```python
from build123d import *

# Parameters (mm, degrees)
F0_R     = 2.0955
F1_DEPTH = 6.35
F5_D     = 2.2606
F5_DEPTH = 5.08
F5_START = 0.1014065
F5_TIP   = 0.6791527577


with BuildPart() as f1:
    # F0 (on Top) → F1 (new body)
    with BuildSketch(Plane.XY):
        with BuildLine():
            ThreePointArc((-6.3375855209, 0.396875), (-0.1985345593, -6.3468956214), (6.35, 0))
            ThreePointArc((6.35, 0), (6.3468956214, 0.1985345593), (6.3375855209, 0.396875))
            ThreePointArc((6.3375855209, 0.396875), (0, 6.35), (-6.3375855209, 0.396875))
        make_face()
        Circle(F0_R, mode=Mode.SUBTRACT)
        with BuildLine():
            ThreePointArc((-6.3375855209, 0.396875), (0, 6.35), (6.3375855209, 0.396875))
            Line((6.3375855209, 0.396875), (0, 101.6))
            Line((0, 101.6), (-6.3375855209, 0.396875))
        make_face()
    extrude(amount=F1_DEPTH)

    # F5
    # its depths count from where the whole tool has entered the part; down to there all is cleared
    with Locations(Plane.XZ.offset(6.35).offset(-F5_START)):
        with Locations((0, 3.175)):
            Hole(F5_D / 2, depth=F5_DEPTH)
            with Locations((0, 0, -(F5_DEPTH + F5_TIP / 2))):  # 118° drill point
                Cone(0, F5_D / 2, F5_TIP, mode=Mode.SUBTRACT)


solid = f1.part
```
Geometry: final body of the model. Coordinates: model frame, mm. Coordinates: 2 decimals unless noted, no trailing zeros. Order: outer loops, then holes, each group sorted by start corner. A loop starts at its lowest first (then second) coordinate and runs counter-clockwise, first axis right, second up. Notation, with made-up numbers: (9, 89) -> (41, 89) arc R29 ccw to (41, 111) -> close; hole circle Ø5 at (12, -7). An arc over 180 degrees is marked (long way). Answer in a Markdown table with one row per item.
Item 1: Section B-B on x = 4.75. Output: boundary loops of the cut face in (y, z), plus the area to 3 significant figures.
Return value:
| item | result |
|---|---|
| outline | (-4.21, 0) -> (25.75, 0) -> (25.75, 6.35) -> (-4.21, 6.35) -> close |
| area | 190 mm² |
Item 2: Draft query along X for faces 1 (the flat face through (0, 36, 0)), 2 (the flat face through (3.213, 50.29, 3.131)), 3 (the flat face through (-3.124, 51.707, 3.131)), 4 (the cylindrical face through (1.13, -4.03, 3.22)). Return one class per face: released by +X, released by -X, zero draft, split by the parting line, or undercut.
Return value:
| item | result |
|---|---|
| face 1 | zero draft |
| face 2 | released by +X |
| face 3 | released by -X |
| face 4 | undercut |
Item 3: Contact query for flat-ended pins moving along their axis: P1, Ø5, axis at x = -3.5, y = 52.5, coming from the -Z side; P2, Ø1.4, axis at x = 0, z = 3.175, coming from the -Y side. Output: stop coordinate, or through.
Return value:
| item | result |
|---|---|
| P1 | stops at z = 0 |
| P2 | stops at y = 1.98 |
Item 4: Ray query, L1, parallel to X at y = 15.5, z = 0.5; L2, parallel to X at y = 18, z = 1.75. Return the intervals inside material, ascending.
Return value:
| item | result |
|---|---|
| L1 | x = -5.39 to 5.39 |
| L2 | x = -5.24 to 5.24 |
Item 5: Section A-A on y = 28.5. Output: boundary loops of the cut face in (x, z), plus the area to 3 significant figures.
Return value:
| item | result |
|---|---|
| outline | (-4.58, 0) -> (4.58, 0) -> (4.58, 6.35) -> (-4.58, 6.35) -> close |
| area | 58.1 mm² |
